```python
from build123d import *

# Parameters (mm, degrees)
SKETCH1_W           = 75
SKETCH1_H           = 50
BOSS_EXTRUDE1_DEPTH = 12
SKETCH2_R           = 14.01
CUT_EXTRUDE1_DEPTH  = 12
SKETCH9_R           = 2
CUT_EXTRUDE2_DEPTH  = 19


with BuildPart() as part:
    # Sketch1 → Boss-Extrude1 (new body)
    with BuildSketch(Plane(origin=(0, 0, 0), x_dir=(1, 0, 0), z_dir=(0, 1, 0))):
        Rectangle(SKETCH1_W, SKETCH1_H)
    extrude(amount=BOSS_EXTRUDE1_DEPTH)

    # Sketch2 → Cut-Extrude1 (cut)
    with BuildSketch(Plane(origin=(0, 12, 0), x_dir=(1, 0, 0), z_dir=(0, 1, 0))):
        with Locations(Location((0, 0, 0), (0, 0, 270))):
            Circle(SKETCH2_R)
    extrude(amount=-CUT_EXTRUDE1_DEPTH, mode=Mode.SUBTRACT)

    # Sketch9 → Cut-Extrude2 (cut)
    with BuildSketch(Plane.XZ):
        with Locations(Location((-9.886968549, 16.388822862, 0), (0, 0, 270))):
            Circle(SKETCH9_R)
        with Locations(Location((9.886968549, 16.388822862, 0), (0, 0, 90))):
            Circle(SKETCH9_R)
        with Locations(Location((-9.886968549, -16.388822862, 0), (0, 0, 90))):
            Circle(SKETCH9_R)
        with Locations(Location((9.886968549, -16.388822862, 0), (0, 0, 270))):
            Circle(SKETCH9_R)
    extrude(amount=-CUT_EXTRUDE2_DEPTH, mode=Mode.SUBTRACT)

    # Sketch11 → Ø5.0mm Dowel Hole1 (revolve, cut)
    with BuildSketch(Plane(origin=(20, 6, -25), x_dir=(0, 1, 0), z_dir=(1, 0, 0))):
        Polygon((0, 0), (0, 51.502151548), (2.5, 50), (2.5, 0), align=None)
    f_5_0mm_dowel_hole1 = revolve(axis=Axis((20, 6, -31.35), (0, 0, 1)), mode=Mode.SUBTRACT)

    # Mirror1: Ø5.0mm Dowel Hole1 across plane
    add(f_5_0mm_dowel_hole1.mirror(Plane(origin=(0, 0, 0), x_dir=(0, 0, 1), z_dir=(1, 0, 0))), mode=Mode.SUBTRACT)


solid = part.part
```
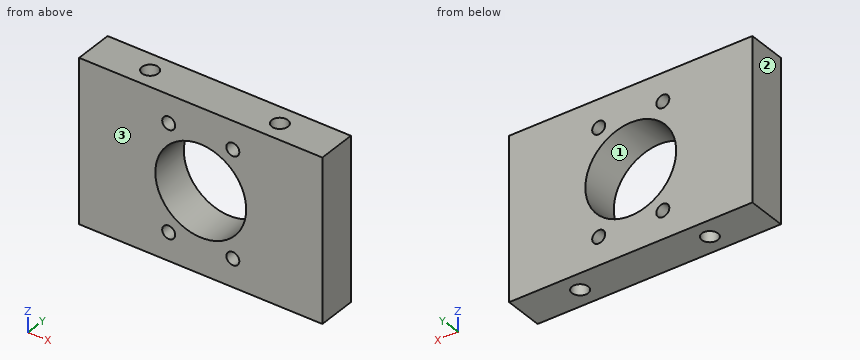
The model under review builds one solid part; all positions refer to its coordinate system, in mm. Face numbers are marked on the shaded views. Round coordinates to 2 decimals unless told otherwise and drop trailing zeros. Order: outer loops, then holes, each group sorted by start corner. A loop starts at its lowest first (then second) coordinate and runs counter-clockwise, first axis right, second up.
Item 1: Add section A-A, the plane z = 0. State the section outline as (x, y) points, and give its area (3 significant figures).
Working result:
outline: (-37.5, 0) - (-14.01, 0) - (-14.01, 12) - (-37.5, 12) - close; (14.01, 0) - (37.5, 0) - (37.5, 12) - (14.01, 12) - close; hole circle Ø5 at (-20, 6); hole circle Ø5 at (20, 6)
area: 524 mm2
Item 2: Add section D-D, the plane x = 20. State the section outline as (y, z) points, and give its area (3 significant figures).
Working result:
outline: (0, -25) - (3.5, -25) - (3.5, 25) - (0, 25) - close; (8.5, -25) - (12, -25) - (12, 25) - (8.5, 25) - close
area: 350 mm2
Item 3: Draft analysis for pull direction X (two halves, no side actions). For the marked faces 1, 2 and 3, state which applies: released by +X, released by -X, zero draft, split by the parting line, or undercut.
Working result:
face 1: undercut
face 2: released by -X
face 3: zero draft
Item 4: To check wall thickness, follow probe 1 along X at (y, z) = (8.25, 7); probe 2 along X at (y, z) = (5.75, 4); probe 3 along Z at (x, y) = (-8.5, 7.75). State the ranges of each line that lie inside material, in increasing order.
Working result:
probe 1: x = -37.5 to -21.09, -18.91 to -12.14, 12.14 to 18.91, 21.09 to 37.5
probe 2: x = -37.5 to -22.49, -17.51 to -13.43, 13.43 to 17.51, 22.49 to 37.5
probe 3: z = -25 to -17.83, -14.95 to -11.14, 11.14 to 14.95, 17.83 to 25
Item 5: Add section C-C, the plane y = 5.5. State the section outline as (x, z) points.
Working result:
outline: (-37.5, -25) - (-22.45, -25) - (-22.45, 25) - (-37.5, 25) - close; (-17.55, -25) - (17.55, -25) - (17.55, 25) - (-17.55, 25) - close; (22.45, -25) - (37.5, -25) - (37.5, 25) - (22.45, 25) - close; hole circle Ø28.02 at (0, 0); hole circle Ø4 at (-9.89, -16.39); hole circle Ø4 at (-9.89, 16.39); hole circle Ø4 at (9.89, -16.39); hole circle Ø4 at (9.89, 16.39)
Item 6: Add section B-B, the plane x = 0. State the section outline as (y, z) points.
Working result:
outline: (0, -25) - (12, -25) - (12, -14.01) - (0, -14.01) - close; (0, 14.01) - (12, 14.01) - (12, 25) - (0, 25) - close
